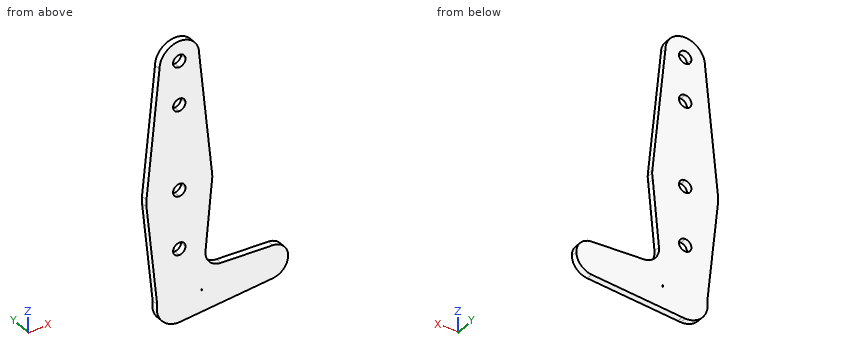
from build123d import *

# Parameters (mm, degrees)
F1_DEPTH = 3.048


with BuildPart() as f1:
    # F0 (on Front) → F1 (new body)
    with BuildSketch(Plane.XZ):
        with BuildLine():
            Line((15.875, 0), (15.5906901587, -2.9909873578))
            ThreePointArc((15.5906901587, -2.9909873578), (15.803762705, -1.5022347903), (15.875, 0))
        make_face()
        with BuildLine():
            Line((1.4003408265, -63.2241331384), (0, -63.3149812557))
            ThreePointArc((0, -63.3149812557), (0.7016423253, -63.2922453786), (1.4003408265, -63.2241331384))
        make_face()
        with BuildLine():
            ThreePointArc((36.5125, -52.4770691991), (39.0220603724, -58.2685610319), (44.9638707463, -60.3979178346))
            ThreePointArc((44.9638707463, -60.3979178346), (50.2414918328, -57.9050088266), (52.3875, -52.4770691991))
            ThreePointArc((52.3875, -52.4770691991), (50.2414918328, -47.0491295715), (44.9638707463, -44.5562205636))
            ThreePointArc((44.9638707463, -44.5562205636), (39.0220603724, -46.6855773663), (36.5125, -52.4770691991))
        make_face()
        with BuildLine():
            Line((12.6191526396, -34.2520619409), (11.8439294246, -42.4075405738))
            Line((11.8439294246, -42.4075405738), (20.0189840628, -42.9379031172))
            ThreePointArc((20.0189840628, -42.9379031172), (14.4819098788, -40.1601346792), (12.6191526396, -34.2520619409))
        make_face()
        with BuildLine():
            ThreePointArc((9.525, 61.8229308009), (0, 71.3479308009), (-9.525, 61.8229308009))
            Line((-9.525, 61.8229308009), (-2.9845, 61.8229308009))
            ThreePointArc((-2.9845, 61.8229308009), (0, 64.8074308009), (2.9845, 61.8229308009))
            ThreePointArc((2.9845, 61.8229308009), (2.1103601885, 59.7125706125), (0, 58.8384308009))
            Line((0, 58.8384308009), (0, 52.2979308009))
            ThreePointArc((0, 52.2979308009), (6.7351920908, 55.0877387101), (9.525, 61.8229308009))
        make_face()
        with BuildLine():
            Line((-2.9845, 61.8229308009), (-9.525, 61.8229308009))
            ThreePointArc((-9.525, 61.8229308009), (-6.7351920908, 55.0877387101), (0, 52.2979308009))
            Line((0, 52.2979308009), (0, 58.8384308009))
            ThreePointArc((0, 58.8384308009), (-2.1103601885, 59.7125706125), (-2.9845, 61.8229308009))
        make_face()
        with BuildLine():
            Line((0, 37.8262675612), (0, 15.875))
            ThreePointArc((0, 15.875), (10.6283048728, 11.7921482577), (15.7896751859, 1.6437099882))
            Line((15.7896751859, 1.6437099882), (9.525, 61.8229308009))
            ThreePointArc((9.525, 61.8229308009), (6.7351920908, 55.0877387101), (0, 52.2979308009))
            Line((0, 52.2979308009), (0, 43.7952675612))
            ThreePointArc((0, 43.7952675612), (2.1103601885, 42.9211277496), (2.9845, 40.8107675612))
            ThreePointArc((2.9845, 40.8107675612), (2.1103601885, 38.7004073727), (0, 37.8262675612))
        make_face()
        with BuildLine():
            Line((-9.525, 61.8229308009), (-15.7896751859, 1.6437099882))
            ThreePointArc((-15.7896751859, 1.6437099882), (-10.6283048728, 11.7921482577), (0, 15.875))
            Line((0, 15.875), (0, 37.8262675612))
            ThreePointArc((0, 37.8262675612), (-2.9845, 40.8107675612), (0, 43.7952675612))
            Line((0, 43.7952675612), (0, 52.2979308009))
            ThreePointArc((0, 52.2979308009), (-6.7351920908, 55.0877387101), (-9.525, 61.8229308009))
        make_face()
        with BuildLine():
            ThreePointArc((-15.7896751859, 1.6437099882), (-15.8749970359, -0.0097010433), (-15.7876544862, -1.6630065613))
            ThreePointArc((-15.7876544862, -1.6630065613), (-10.6210968322, -11.7986408997), (0, -15.875))
            Line((0, -15.875), (0, -2.9845))
            ThreePointArc((0, -2.9845), (-2.9845, 0), (0, 2.9845))
            Line((0, 2.9845), (0, 11.0229308009))
            Line((0, 11.0229308009), (0, 15.875))
            ThreePointArc((0, 15.875), (-10.6283048728, 11.7921482577), (-15.7896751859, 1.6437099882))
        make_face()
        with BuildLine():
            Line((0, -31.1324340047), (0, -41.6391571425))
            ThreePointArc((0, -41.6391571425), (0.7016423253, -41.6618930196), (1.4003408265, -41.7300052598))
            Line((1.4003408265, -41.7300052598), (11.8439294246, -42.4075405738))
            Line((11.8439294246, -42.4075405738), (12.6191526396, -34.2520619409))
            Line((12.6191526396, -34.2520619409), (15.5906901587, -2.9909873578))
            ThreePointArc((15.5906901587, -2.9909873578), (10.1127073698, -12.2371881841), (0, -15.875))
            Line((0, -15.875), (0, -25.1634340047))
            ThreePointArc((0, -25.1634340047), (2.1103601885, -26.0375738162), (2.9845, -28.1479340047))
            ThreePointArc((2.9845, -28.1479340047), (2.1103601885, -30.2582941931), (0, -31.1324340047))
        make_face()
        with BuildLine():
            Line((10.8867652033, -52.4770691991), (10.8379120566, -52.4770691991))
            ThreePointArc((10.8379120566, -52.4770691991), (8.1436204624, -59.6284175691), (1.4003408265, -63.2241331384))
            Line((1.4003408265, -63.2241331384), (44.9638707463, -60.3979178346))
            ThreePointArc((44.9638707463, -60.3979178346), (39.0220603724, -58.2685610319), (36.5125, -52.4770691991))
            Line((36.5125, -52.4770691991), (10.8867652033, -52.4770691991))
        make_face()
        with BuildLine():
            Line((0, -2.9845), (0, -15.875))
            ThreePointArc((0, -15.875), (10.1127073698, -12.2371881841), (15.5906901587, -2.9909873578))
            Line((15.5906901587, -2.9909873578), (15.875, 0))
            ThreePointArc((15.875, 0), (15.8536544458, 0.8229615497), (15.7896751859, 1.6437099882))
            ThreePointArc((15.7896751859, 1.6437099882), (10.6283048728, 11.7921482577), (0, 15.875))
            Line((0, 15.875), (0, 11.0229308009))
            Line((0, 11.0229308009), (0, 2.9845))
            ThreePointArc((0, 2.9845), (2.1103601885, 2.1103601885), (2.9845, 0))
            ThreePointArc((2.9845, 0), (2.1103601885, -2.1103601885), (0, -2.9845))
        make_face()
        with BuildLine():
            Line((0, -52.4770691991), (0, -41.6391571425))
            ThreePointArc((0, -41.6391571425), (-6.9124383958, -44.1297023585), (-10.6479290016, -50.4566866308))
            ThreePointArc((-10.6479290016, -50.4566866308), (-8.3473668405, -59.3895075949), (0, -63.3149812557))
            Line((0, -63.3149812557), (1.4003408265, -63.2241331384))
            ThreePointArc((1.4003408265, -63.2241331384), (8.1436204624, -59.6284175691), (10.8379120566, -52.4770691991))
            Line((10.8379120566, -52.4770691991), (10.6890844764, -52.4770691991))
            Line((10.6890844764, -52.4770691991), (0, -52.4770691991))
        make_face()
        with BuildLine():
            Line((20.0189840628, -42.9379031172), (11.8439294246, -42.4075405738))
            Line((11.8439294246, -42.4075405738), (10.8867652033, -52.4770691991))
            Line((10.8867652033, -52.4770691991), (36.5125, -52.4770691991))
            ThreePointArc((36.5125, -52.4770691991), (39.0220603724, -46.6855773663), (44.9638707463, -44.5562205636))
            Line((44.9638707463, -44.5562205636), (20.0189840628, -42.9379031172))
        make_face()
        with BuildLine():
            Line((11.8439294246, -42.4075405738), (1.4003408265, -41.7300052598))
            ThreePointArc((1.4003408265, -41.7300052598), (7.800803165, -44.9532531642), (10.7906490607, -51.4660149992))
            ThreePointArc((10.7906490607, -51.4660149992), (10.8260898597, -51.9709900586), (10.8379120566, -52.4770691991))
            Line((10.8379120566, -52.4770691991), (10.8867652033, -52.4770691991))
            Line((10.8867652033, -52.4770691991), (11.8439294246, -42.4075405738))
        make_face()
        with BuildLine():
            Line((1.4003408265, -41.7300052598), (0, -41.6391571425))
            Line((0, -41.6391571425), (0, -52.4770691991))
            Line((0, -52.4770691991), (10.6890844764, -52.4770691991))
            Line((10.6890844764, -52.4770691991), (10.7906490607, -51.4660149992))
            ThreePointArc((10.7906490607, -51.4660149992), (7.800803165, -44.9532531642), (1.4003408265, -41.7300052598))
        make_face()
        with BuildLine():
            ThreePointArc((-10.6479290016, -50.4566866308), (-6.9124383958, -44.1297023585), (0, -41.6391571425))
            Line((0, -41.6391571425), (0, -31.1324340047))
            ThreePointArc((0, -31.1324340047), (-2.9845, -28.1479340047), (0, -25.1634340047))
            Line((0, -25.1634340047), (0, -15.875))
            ThreePointArc((0, -15.875), (-10.6210968322, -11.7986408997), (-15.7876544862, -1.6630065613))
            Line((-15.7876544862, -1.6630065613), (-10.6479290016, -50.4566866308))
        make_face()
    extrude(amount=F1_DEPTH)


solid = f1.part
The listing builds one solid part. Answer for the finished solid, in the listing's coordinates (mm). Round coordinates to 2 decimals unless told otherwise and drop trailing zeros. Order: outer loops, then holes, each group sorted by start corner. A loop starts at its lowest first (then second) coordinate and runs counter-clockwise, first axis right, second up. Notation, with made-up numbers: (50, 89.5) -> (55, 89.5) arc R35 ccw to (55, 127.5) -> close; hole circle Ø4 at (16, 83). An arc over 180 degrees is marked (long way). One line per item, written item: value.
Item 1: Find section C-C, the plane z = -9. Give the vertices of the cut face in (x, y).
Taken from the geometry:
outline: (-15.01, -3.05) -> (15.02, -3.05) -> (15.02, 0) -> (-15.01, 0) -> close
Item 2: Find section A-A, the plane y = -2.05. State how many separate pieces and enclosed holes the cut face has, then the cut area to 3 significant figures.
Taken from the geometry:
separate pieces: 1
enclosed holes: 6
area: 3,920 mm2
Item 3: Straight lines are drawn through the part: L1, parallel to Z at x = 2, y = -2.55; L2, parallel to X at y = -1.25, z = -27.5; L3, parallel to X at y = -2.6, z = 61.5. For each, find the intervals that lie inside material, in ascending order.
Taken from the geometry:
L1: z = -63.19 to -30.36, -25.93 to -2.22, 2.22 to 38.6, 43.03 to 59.61, 64.04 to 71.14
L2: x = -13.07 to -2.91, 2.91 to 13.26
L3: x = -9.56 to -2.97, 2.97 to 9.56
Item 4: Given P1, Ø12, axis at x = -6, z = 52.5, coming from the +Y side; P2, Ø1.5, axis at y = -2.5, z = -2, coming from the +X side, each flat-ended and moving along its own axis, determine where each tip first touches the part or whether it passes through.
Taken from the geometry:
P1: stops at y = 0
P2: stops at x = 15.83
Item 5: Find section B-B, the plane x = 48.5. Give the vertices of the cut face in (y, z).
Taken from the geometry:
outline: (-3.05, -59.3) -> (0, -59.3) -> (0, -45.65) -> (-3.05, -45.65) -> close
